Model file for the job. Use its own axes, mm. A direction names the side the tool comes from. Coordinates: 2 decimals unless noted, no trailing zeros. Write each loop counter-clockwise with the first axis right and the second up, starting at its lowest first coordinate (ties: lowest second). Pieces come first, ordered by that corner, then holes.
Q1. Band-saw the part on B-B, the plane y = 0. State how many separate pieces and enclosed holes the cut face has, plus the area to 3 significant figures.
Q2. Pin check, flat tips, straight feed: P1, Ø5, axis at y = 35.5, z = 54.5, coming from the -X side; P2, Ø12, axis at x = -3, z = -15.5, coming from the +Y side; P3, Ø12, axis at y = 60, z = -30.5, coming from the -X side; P4, Ø6, axis at y = 43, z = 82.5, coming from the -X side. Stop position of each tip, or through.
Q3. Pull direction Y, two halves, no side cores. Call faces 1 (the flat face through (-28, 55, 109)), 2 (the flat face through (0, 63, 13)), 3 (the flat face through (-27, -1, -79)): released by +Y, released by -Y, zero draft, split by the parting line, or undercut.
Q4. Band-saw the part on A-A, the plane x = -42. Write the cut outline in (y, z), plus the area to 3 significant figures.
Q5. Band-saw the part on D-D, the plane z = -7.5. Write the cut outline in (x, y), plus the area to 3 significant figures.
Q6. Which spindle directions (+Z, -Z, +X, -X, +Y, -Y) get a long thin tool onto all of the face, cutting with end or side? Do faces 4 (the flat face through (-53, -43, 86.5)), 5 (the flat face through (13, 0, -84)), 6 (the flat face through (-30, 1, 133)), 7 (the flat face through (-68, 0, -85)). Say none if no direction does.
Q7. Band-saw the part on C-C, the plane x = 34.5. Write the cut outline in (y, z), plus the area to 3 significant figures.
Q8. Drill centre lines: probe 1 along Y at (x, z) = (-53.95, 82.5); probe 2 along Y at (x, z) = (9, -84.25); probe 3 along Y at (x, z) = (36, -40.5). Where is each one in solid material? Low to high.
from build123d import *

# Parameters (mm, degrees)
SKETCH1_W                = 238
SKETCH1_H                = 152
SKETCH1_W_2              = 158
SKETCH1_H_2              = 122
BOSS_EXTRUDE1_DEPTH      = 50
SKETCH4_W                = 158
SKETCH4_H                = 122
BOSS_EXTRUDE2_DEPTH      = 10
CUT_EXTRUDE1_START       = -30
SKETCH5_W                = 8
SKETCH5_H                = 132
CUT_EXTRUDE1_DEPTH       = 204
SKETCH8_W                = 25
SKETCH8_H                = 152
CUT_EXTRUDE3_DEPTH       = 50
SKETCH11_W               = 15
SKETCH11_H               = 30
BOSS_EXTRUDE4_DEPTH      = 75
SKETCH16_W               = 15
SKETCH16_H               = 30
BOSS_EXTRUDE6_DEPTH      = 5
SKETCH18_R               = 4
SKETCH18_W               = 8
SKETCH18_H               = 5
CUT_EXTRUDE8_DEPTH       = 7.5
SKETCH19_R               = 2
CUT_EXTRUDE9_DEPTH       = 10
SKETCH20_W               = 50
SKETCH20_H               = 152
BOSS_EXTRUDE7_DEPTH      = 20
SKETCH21_W               = 60
SKETCH21_H               = 110
BOSS_EXTRUDE8_DEPTH      = 56
SKETCH22_W               = 50
SKETCH22_H               = 95
CUT_EXTRUDE10_DEPTH      = 54
SKETCH24_R               = 2.75
CUT_EXTRUDE11_DEPTH      = 1
CUT_EXTRUDE11_DEPTH_BACK = 40
SKETCH25_W               = 7
SKETCH25_H               = 65
CUT_EXTRUDE12_DEPTH      = 12
SKETCH26_W               = 52.5
SKETCH26_H               = 6
CUT_EXTRUDE13_DEPTH      = 40
SKETCH27_W               = 15
SKETCH27_H               = 83
CUT_EXTRUDE14_DEPTH      = 30
SKETCH29_R               = 9.5
CUT_EXTRUDE15_DEPTH      = 6
SKETCH30_R               = 2.5
CUT_EXTRUDE16_DEPTH      = 6
SKETCH34_W               = 45
SKETCH34_H               = 10
CUT_EXTRUDE17_DEPTH      = 10


with BuildPart() as part:
    # Sketch1 → Boss-Extrude1 (new body)
    with BuildSketch(Plane(origin=(0, 0, 0), x_dir=(0, 0, -1), z_dir=(1, 0, 0))):
        Rectangle(SKETCH1_W, SKETCH1_H)
        Rectangle(SKETCH1_W_2, SKETCH1_H_2, mode=Mode.SUBTRACT)
    extrude(amount=BOSS_EXTRUDE1_DEPTH)

    # Sketch4 → Boss-Extrude2 (add)
    with BuildSketch(Plane(origin=(50, 0, 0), x_dir=(0, 0, -1), z_dir=(1, 0, 0))):
        Rectangle(SKETCH4_W, SKETCH4_H)
    extrude(amount=-BOSS_EXTRUDE2_DEPTH)

    # Sketch5 → Cut-Extrude1 (cut)
    with BuildSketch(Plane.XY.offset(119).offset(CUT_EXTRUDE1_START)):
        with Locations((9, 0)):
            Rectangle(SKETCH5_W, SKETCH5_H)
    extrude(amount=-CUT_EXTRUDE1_DEPTH, mode=Mode.SUBTRACT)

    # Sketch8 → Cut-Extrude3 (cut)
    with BuildSketch(Plane.ZY):
        with Locations((-106.5, 0)):
            Rectangle(SKETCH8_W, SKETCH8_H)
    extrude(amount=-CUT_EXTRUDE3_DEPTH, mode=Mode.SUBTRACT)

    # Sketch11 → Boss-Extrude4 (add)
    with BuildSketch(Plane.ZY):
        with Locations((-86.5, 0)):
            Rectangle(SKETCH11_W, SKETCH11_H)
    extrude(amount=BOSS_EXTRUDE4_DEPTH)

    # Sketch16 → Boss-Extrude6 (add)
    with BuildSketch(Plane.ZY.offset(75)):
        with Locations((-86.5, 0)):
            Rectangle(SKETCH16_W, SKETCH16_H)
    extrude(amount=BOSS_EXTRUDE6_DEPTH)

    # Sketch18 → Cut-Extrude8 (cut)
    with BuildSketch(Plane(origin=(0, 0, -94), x_dir=(-1, 0, 0), z_dir=(0, 0, -1))):
        with Locations((-9, 71)):
            Circle(SKETCH18_R)
        with Locations((-9, -71)):
            Circle(SKETCH18_R)
        with Locations((-9, 68.5)):
            Rectangle(SKETCH18_W, SKETCH18_H)
        with Locations((-9, -68.5)):
            Rectangle(SKETCH18_W, SKETCH18_H)
    extrude(amount=-CUT_EXTRUDE8_DEPTH, mode=Mode.SUBTRACT)

    # Sketch19 → Cut-Extrude9 (cut)
    with BuildSketch(Plane(origin=(0, 0, -86.5), x_dir=(-1, 0, 0), z_dir=(0, 0, -1))):
        with Locations((-9, 71)):
            Circle(SKETCH19_R)
        with Locations((-9, -71)):
            Circle(SKETCH19_R)
    extrude(amount=-CUT_EXTRUDE9_DEPTH, mode=Mode.SUBTRACT)

    # Sketch20 → Boss-Extrude7 (add)
    with BuildSketch(Plane.XY.offset(119)):
        with Locations((25, 0)):
            Rectangle(SKETCH20_W, SKETCH20_H)
    extrude(amount=BOSS_EXTRUDE7_DEPTH)

    # Sketch21 → Boss-Extrude8 (add)
    with BuildSketch(Plane.ZY):
        with Locations((109, 0)):
            Rectangle(SKETCH21_W, SKETCH21_H)
    extrude(amount=BOSS_EXTRUDE8_DEPTH)

    # Sketch22 → Cut-Extrude10 (cut)
    with BuildSketch(Plane(origin=(0, 0, 79), x_dir=(-1, 0, 0), z_dir=(0, 0, -1))):
        with Locations((25, 0)):
            Rectangle(SKETCH22_W, SKETCH22_H)
    extrude(amount=-CUT_EXTRUDE10_DEPTH, mode=Mode.SUBTRACT)

    # Sketch24 → Cut-Extrude11 (cut, two sides)
    with BuildSketch(Plane.ZY) as cut_extrude11_sk:
        with Locations((108.6, 36)):
            Circle(SKETCH24_R)
        with Locations((108.6, -36)):
            Circle(SKETCH24_R)
    extrude(amount=CUT_EXTRUDE11_DEPTH, mode=Mode.SUBTRACT)
    extrude(cut_extrude11_sk.sketch, amount=-CUT_EXTRUDE11_DEPTH_BACK, mode=Mode.SUBTRACT)

    # Sketch25 → Cut-Extrude12 (cut)
    with BuildSketch(Plane(origin=(0, 0, 133), x_dir=(-1, 0, 0), z_dir=(0, 0, -1))):
        with Locations((21.5, 0)):
            Rectangle(SKETCH25_W, SKETCH25_H)
    extrude(amount=-CUT_EXTRUDE12_DEPTH, mode=Mode.SUBTRACT)

    # Sketch26 → Cut-Extrude13 (cut)
    with BuildSketch(Plane.ZY):
        with Locations((105.25, 44.5)):
            Rectangle(SKETCH26_W, SKETCH26_H)
        with Locations((105.25, -44.5)):
            Rectangle(SKETCH26_W, SKETCH26_H)
    extrude(amount=-CUT_EXTRUDE13_DEPTH, mode=Mode.SUBTRACT)

    # Sketch27 → Cut-Extrude14 (cut)
    with BuildSketch(Plane.ZY.offset(-13)):
        with Locations((86.5, 0)):
            Rectangle(SKETCH27_W, SKETCH27_H)
    extrude(amount=-CUT_EXTRUDE14_DEPTH, mode=Mode.SUBTRACT)

    # Sketch29 → Cut-Extrude15 (cut)
    with BuildSketch(Plane.XY.offset(-79)):
        with Locations((-67.5, 0)):
            Circle(SKETCH29_R)
    extrude(amount=-CUT_EXTRUDE15_DEPTH, mode=Mode.SUBTRACT)

    # Sketch30 → Cut-Extrude16 (cut)
    with BuildSketch(Plane.ZY.offset(56)):
        with Locations((82.5, 8)):
            Circle(SKETCH30_R)
        with Locations((107.5, 8)):
            Circle(SKETCH30_R)
        with Locations((82.5, 43)):
            Circle(SKETCH30_R)
        with Locations((107.5, 43)):
            Circle(SKETCH30_R)
    extrude(amount=-CUT_EXTRUDE16_DEPTH, mode=Mode.SUBTRACT)

    # Sketch34 → Cut-Extrude17 (cut)
    with BuildSketch(Plane.ZY.offset(56)):
        with Locations((109, -42.5)):
            Rectangle(SKETCH34_W, SKETCH34_H)
    extrude(amount=-CUT_EXTRUDE17_DEPTH, mode=Mode.SUBTRACT)


solid = part.part
Answer sheet:
1. separate pieces: 3
1. enclosed holes: 0
1. area: 6,380 mm2
2. P1: stops at x = 40
2. P2: stops at y = 76
2. P3: stops at x = 0
2. P4: stops at x = -56
3. face 1: released by +Y
3. face 2: zero draft
3. face 3: undercut
4. outline: (-55, 79) - (-47.5, 79) - (-47.5, 133) - (47.5, 133) - (47.5, 79) - (55, 79) - (55, 139) - (-55, 139) - close; (-15, -94) - (15, -94) - (15, -79) - (-15, -79) - close
4. area: 1,920 mm2
5. outline: (0, -76) - (50, -76) - (50, 76) - (0, 76) - (0, 61) - (5, 61) - (5, 66) - (13, 66) - (13, 61) - (40, 61) - (40, -61) - (13, -61) - (13, -66) - (5, -66) - (5, -61) - (0, -61) - close
5. area: 2,640 mm2
6. face 4: -X
6. face 5: -Z
6. face 6: none
6. face 7: +Z
7. outline: (-76, -94) - (76, -94) - (76, 139) - (-76, 139) - close; hole (-61, -79) - (61, -79) - (61, 79) - (47.5, 79) - (47.5, 131.5) - (41.5, 131.5) - (41.5, 94) - (-41.5, 94) - (-41.5, 131.5) - (-47.5, 131.5) - (-47.5, 79) - (-61, 79) - close; hole circle Ø5.5 at (-36, 108.6); hole circle Ø5.5 at (36, 108.6)
7. area: 14,200 mm2
8. probe 1: y = -55 to 5.5, 10.5 to 40.5, 45.5 to 55
8. probe 2: y = -76 to -73, -69 to -66, 66 to 69, 73 to 76
8. probe 3: y = -76 to -61, 61 to 76
